from build123d import *

# Parameters (mm, degrees)
SKETCH_1_R          = 14.25
SKETCH_1_R_2        = 12.4
EXTRUDE_1_DEPTH     = 11.5
EXTRUDE_START       = 2
SKETCH_2_R          = 14.25
SKETCH_2_R_2        = 4.5
SKETCH_2_R_3        = 1.5
EXTRUDE_2_DEPTH     = 2
SKETCH_4_W          = 16.5
SKETCH_4_H          = 7.711801842
CUT_EXTRUDE_2_DEPTH = 19
EXTRUDE_START_2     = -3
SKETCH_5_R          = 1.5
SKETCH_5_R_2        = 2.058377943
EXTRUDE_3_DEPTH     = 3
FILLET_1_R          = 5


with BuildPart() as part:
    # 草图1 → 凸台-拉伸1 (new body)
    with BuildSketch(Plane.XY):
        Circle(SKETCH_1_R)
        Circle(SKETCH_1_R_2, mode=Mode.SUBTRACT)
    extrude(amount=EXTRUDE_1_DEPTH)

    # 草图2 → 凸台-拉伸2 (add)
    with BuildSketch(Plane(origin=(0, 0, 0), x_dir=(-1, 0, 0), z_dir=(0, 0, -1)).offset(EXTRUDE_START)):
        Circle(SKETCH_2_R)
        Circle(SKETCH_2_R_2, mode=Mode.SUBTRACT)
        with Locations((-10, 0)):
            Circle(SKETCH_2_R_3, mode=Mode.SUBTRACT)
    extrude(amount=-EXTRUDE_2_DEPTH)

    # 草图4 → 切除-拉伸2 (cut)
    with BuildSketch(Plane.XY.offset(11.5)):
        with Locations((0, -12.4)):
            Rectangle(SKETCH_4_W, SKETCH_4_H)
    extrude(amount=-CUT_EXTRUDE_2_DEPTH, mode=Mode.SUBTRACT)

    # 草图5 → 凸台-拉伸3 (add)
    # profile 1 of 2: a face of its own
    with BuildSketch(Plane.XY.offset(11.5).offset(EXTRUDE_START_2)):
        with BuildLine():
            Line((-24, 4), (-13.677079367, 4))
            ThreePointArc((-13.677079367, 4), (-14.25, 0), (-13.677079367, -4))
            Line((-13.677079367, -4), (-24, -4))
            ThreePointArc((-24, -4), (-28, 0), (-24, 4))
        make_face()
        with Locations((-24, 0)):
            Circle(SKETCH_5_R, mode=Mode.SUBTRACT)
    # profile 2 of 2: a face of its own
    with BuildSketch(Plane.XY.offset(11.5).offset(EXTRUDE_START_2)):
        with BuildLine():
            Line((13.677079367, 4), (24, 4))
            ThreePointArc((24, 4), (28, 0), (24, -4))
            Line((24, -4), (13.677079367, -4))
            ThreePointArc((13.677079367, -4), (14.25, 0), (13.677079367, 4))
        make_face()
        with Locations((24, 0)):
            Circle(SKETCH_5_R_2, mode=Mode.SUBTRACT)
    extrude(amount=EXTRUDE_3_DEPTH)

    # 圆角1
    fillet_1_edges = [part.edges().sort_by_distance(p)[0] for p in [
        (-13.677079367, 4, 10),
        (-13.677079367, -4, 10),
        (-14.25, 0, 8.5),
        (13.677079367, -4, 10),
        (13.677079367, 4, 10),
        (14.25, 0, 8.5),
    ]]
    fillet(fillet_1_edges, radius=FILLET_1_R)


solid = part.part
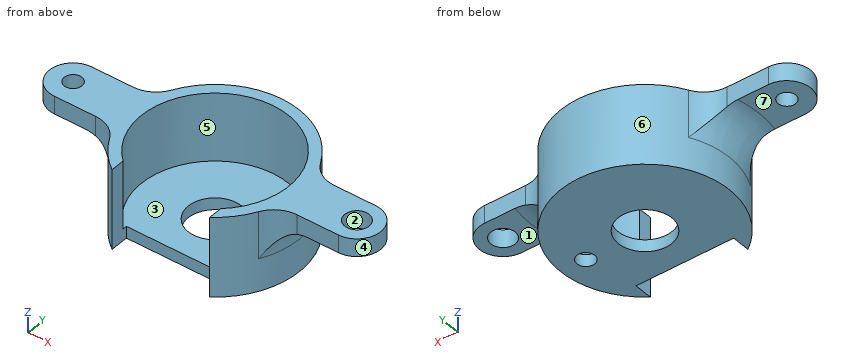
Check sheet for the modelled part. Datum: model origin and axes. Units: mm. Face numbers are marked on the shaded views. A direction names the side the tool comes from. Give positions to 0.01 mm unless a question says otherwise; leave off trailing zeros. Write each loop counter-clockwise with the first axis right and the second up, starting at its lowest first coordinate (ties: lowest second). Pieces come first, ordered by that corner, then holes. Notation, with made-up numbers: (-19, 45.5) -> (32, 45.5) arc R24 ccw to (32, 63.5) -> close; hole circle Ø6 at (-4.75, 72). An arc over 180 degrees is marked (long way). Write item = value, one per line.
Item 1: Release check for a two-part mould opening along X. For the marked faces 1, 2, 3 and 4 record: +X half, -X half, draft (parallel to the pull), parting line (faces both ways), or undercut.
Output:
face_1 = draft
face_2 = undercut
face_3 = undercut
face_4 = +X half
Item 2: Sectioned sample at D-D on x = 10. Record the boundary of the cut face in (y, z), and give its area (3 significant figures).
Output:
outline = (-10.15, -2) -> (-1.5, -2) -> (-1.5, 0) -> (-7.33, 0) -> (-7.33, 11.5) -> (-10.15, 11.5) -> close; (1.5, -2) -> (10.15, -2) -> (10.15, 11.5) -> (7.33, 11.5) -> (7.33, 0) -> (1.5, 0) -> close
area = 99.5 mm^2
Item 3: Sectioned sample at C-C on z = 10. Record the boundary of the cut face in (x, y), and give its area (3 significant figures).
Output:
outline = (-24, -4) -> (-17.02, -4) arc R5 cw to (-12.6, -6.66) arc R14.25 ccw to (-8.25, -11.62) -> (-8.25, -9.26) arc R12.4 cw (long way) to (8.25, -9.26) -> (8.25, -11.62) arc R14.25 ccw to (12.6, -6.66) arc R5 cw to (17.02, -4) -> (24, -4) arc R4 ccw to (24, 4) -> (17.02, 4) arc R5 cw to (12.6, 6.66) arc R14.25 ccw to (-12.6, 6.66) arc R5 cw to (-17.02, 4) -> (-24, 4) arc R4 ccw to start; hole circle Ø3 at (-24, 0); hole circle Ø4.12 at (24, 0)
area = 318 mm^2
Item 4: Scan lines: probe 1 along Y at (x, z) = (24, 9.5); probe 2 along Z at (x, y) = (-4, -5.5); probe 3 along X at (y, z) = (1, 4.75). Record each from-to range of solid material in increasing order. Write a range as from..to.
Output:
probe_1 = -4..-2.06, 2.06..4
probe_2 = -2..0
probe_3 = -14.37..-12.36, 12.36..14.37
Item 5: Tool access check on the marked faces 5, 6 and 7. Record the directions out of +Z, -Z, +X, -X, +Y, -Y that give a thin tool (end or side, any length) a straight path to the whole face; none if there is none.
Output:
face_5 = +Z
face_6 = -Z
face_7 = -Z, -X, +Y, -Y
Item 6: Sectioned sample at A-A on x = 0. Record the boundary of the cut face in (y, z), and give its area (3 significant figures).
Output:
outline = (-8.54, -2) -> (-4.5, -2) -> (-4.5, 0) -> (-8.54, 0) -> close; (4.5, -2) -> (14.25, -2) -> (14.25, 11.5) -> (12.4, 11.5) -> (12.4, 0) -> (4.5, 0) -> close
area = 48.9 mm^2
Item 7: Gauge pin test, flat ends, axial feed: pin 1 (1.5 mm diameter, centred on y = -10, z = 7.5, fed in from -X); pin 2 (2 mm diameter, centred on y = -8, z = 4.5, fed in from +X); pin 3 (3 mm diameter, centred on x = 20, z = 9.5, fed in from +Y); pin 4 (8 mm diameter, centred on x = -4, z = 8, fed in from +Y). Record the tip position at first contact, or that the pin passes through.
Output:
pin_1 = -10.84
pin_2 = 12.41
pin_3 = 4
pin_4 = 14.25
Item 8: Sectioned sample at B-B on y = 0. Count the separate pieces of the cut face and the enclosed holes in it, and give its area (3 significant figures).
Output:
separate_pieces = 5
enclosed_holes = 0
area = 147 mm^2
